```python
from build123d import *

# Parameters (mm, degrees)
SKETCH1_R                    = 3.429
BOSS_EXTRUDE1_DEPTH          = 165.1
SKETCH2_W                    = 12.954
SKETCH2_H                    = 12.954
CUT_EXTRUDE1_DEPTH           = 6.35
CUT_EXTRUDE1_DRAFT           = -45
CUT_EXTRUDE1_PROFILE_2_DEPTH = 6.35
CUT_EXTRUDE1_PROFILE_2_DRAFT = -45
CUT_EXTRUDE1_PROFILE_3_DEPTH = 6.35
CUT_EXTRUDE1_PROFILE_3_DRAFT = -45
SKETCH3_W                    = 6.35
SKETCH3_H                    = 12.7
CUT_EXTRUDE2_DEPTH           = 1.651


with BuildPart() as part:
    # Sketch1 → Boss-Extrude1 (new body)
    with BuildSketch(Plane.XY):
        with BuildLine():
            Line((-49.2125, 0), (-74.6125, 0))
            Line((-74.6125, 0), (-74.6125, -76.2))
            Line((-74.6125, -76.2), (74.6125, -76.2))
            Line((74.6125, -76.2), (74.6125, 0))
            Line((74.6125, 0), (49.2125, 0))
            ThreePointArc((49.2125, 0), (0, -49.2125), (-49.2125, 0))
        make_face()
        with Locations((-55.5625, -57.15)):
            Circle(SKETCH1_R, mode=Mode.SUBTRACT)
        with Locations((55.5625, -57.15)):
            Circle(SKETCH1_R, mode=Mode.SUBTRACT)
    extrude(amount=BOSS_EXTRUDE1_DEPTH)


with BuildPart() as cut_extrude1_tool:
    # Sketch2 → Cut-Extrude1 (with draft: the straight prism first)
    with BuildSketch(Plane(origin=(0, 0, 0), x_dir=(-1, 0, 0), z_dir=(0, 0, -1))):
        with Locations((-61.9125, -19.05)):
            Rectangle(SKETCH2_W, SKETCH2_H)
    extrude(amount=-CUT_EXTRUDE1_DEPTH)
    # Cut-Extrude1: the draft: its side faces are tilted about the plane it starts from
    cut_extrude1_sides = [cut_extrude1_tool.faces().sort_by_distance(p)[0] for p in [
        (68.3895, -19.05, 3.175),
        (61.9125, -25.527, 3.175),
        (55.4355, -19.05, 3.175),
        (61.9125, -12.573, 3.175),
    ]]
    draft(cut_extrude1_sides, Plane(origin=(0, 0, 0), x_dir=(-1, 0, 0), z_dir=(0, 0, -1)), CUT_EXTRUDE1_DRAFT)


with BuildPart() as part_1:
    add(part.part)

    # Cut-Extrude1: cut by cut_extrude1_tool
    add(cut_extrude1_tool.part, mode=Mode.SUBTRACT)


with BuildPart() as cut_extrude1_profile_2_tool:
    # Sketch2 → Cut-Extrude1 profile 2 (with draft: the straight prism first)
    with BuildSketch(Plane(origin=(0, 0, 0), x_dir=(-1, 0, 0), z_dir=(0, 0, -1))):
        with Locations((0, -63.5)):
            Rectangle(SKETCH2_W, SKETCH2_H)
    extrude(amount=-CUT_EXTRUDE1_PROFILE_2_DEPTH)
    # Cut-Extrude1 profile 2: the draft: its side faces are tilted about the plane it starts from
    cut_extrude1_profile_2_sides = [cut_extrude1_profile_2_tool.faces().sort_by_distance(p)[0] for p in [
        (6.477, -63.5, 3.175),
        (0, -69.977, 3.175),
        (-6.477, -63.5, 3.175),
        (0, -57.023, 3.175),
    ]]
    draft(cut_extrude1_profile_2_sides, Plane(origin=(0, 0, 0), x_dir=(-1, 0, 0), z_dir=(0, 0, -1)), CUT_EXTRUDE1_PROFILE_2_DRAFT)


with BuildPart() as part_2:
    add(part_1.part)

    # Cut-Extrude1 profile 2: cut by cut_extrude1_profile_2_tool
    add(cut_extrude1_profile_2_tool.part, mode=Mode.SUBTRACT)


with BuildPart() as cut_extrude1_profile_3_tool:
    # Sketch2 → Cut-Extrude1 profile 3 (with draft: the straight prism first)
    with BuildSketch(Plane(origin=(0, 0, 0), x_dir=(-1, 0, 0), z_dir=(0, 0, -1))):
        with Locations((61.9125, -19.05)):
            Rectangle(SKETCH2_W, SKETCH2_H)
    extrude(amount=-CUT_EXTRUDE1_PROFILE_3_DEPTH)
    # Cut-Extrude1 profile 3: the draft: its side faces are tilted about the plane it starts from
    cut_extrude1_profile_3_sides = [cut_extrude1_profile_3_tool.faces().sort_by_distance(p)[0] for p in [
        (-55.4355, -19.05, 3.175),
        (-61.9125, -25.527, 3.175),
        (-68.3895, -19.05, 3.175),
        (-61.9125, -12.573, 3.175),
    ]]
    draft(cut_extrude1_profile_3_sides, Plane(origin=(0, 0, 0), x_dir=(-1, 0, 0), z_dir=(0, 0, -1)), CUT_EXTRUDE1_PROFILE_3_DRAFT)


with BuildPart() as part_3:
    add(part_2.part)

    # Cut-Extrude1 profile 3: cut by cut_extrude1_profile_3_tool
    add(cut_extrude1_profile_3_tool.part, mode=Mode.SUBTRACT)

    # Sketch3 → Cut-Extrude2 (cut)
    with BuildSketch(Plane(origin=(0, 0, 0), x_dir=(1, 0, 0), z_dir=(0, 1, 0))):
        with Locations((71.4375, -19.05)):
            Rectangle(SKETCH3_W, SKETCH3_H)
        with Locations((71.4375, -57.15)):
            Rectangle(SKETCH3_W, SKETCH3_H)
        with Locations((71.4375, -95.25)):
            Rectangle(SKETCH3_W, SKETCH3_H)
        with Locations((71.4375, -133.35)):
            Rectangle(SKETCH3_W, SKETCH3_H)
        with Locations((-71.4375, -57.15)):
            Rectangle(SKETCH3_W, SKETCH3_H)
        with Locations((-71.4375, -95.25)):
            Rectangle(SKETCH3_W, SKETCH3_H)
        with Locations((-71.4375, -133.35)):
            Rectangle(SKETCH3_W, SKETCH3_H)
        with Locations((-71.4375, -19.05)):
            Rectangle(SKETCH3_W, SKETCH3_H)
    extrude(amount=-CUT_EXTRUDE2_DEPTH, mode=Mode.SUBTRACT)


solid = part_3.part
```
Can you work these out from the model? Positions are in its coordinate system, mm. A direction names the side the tool comes from. Coordinates: 2 decimals unless noted, no trailing zeros. Loops run counter-clockwise (first coordinate to the right, second up) from the corner with the lowest first, then second, coordinate; pieces in that order, holes last. Notation, with made-up numbers: (74.5, -32.75) -> (130.5, -32.75) arc R21 cw to (130.5, -11.75) -> close; hole circle Ø6 at (-37.5, 75.25). An arc over 180 degrees is marked (long way). Put each result on its own line as item: value. Start each with the question number.
Q1. I'm going to push flat-ended pins straight in: P1, Ø3, axis at x = -71.5, z = 21, coming from the +Y side; P2, Ø0.5, axis at y = -0.5, z = 136.5, coming from the +X side; P3, Ø3, axis at x = -44, y = -13, coming from the -Z side; P4, Ø8, axis at x = 30, z = 145, coming from the +Y side. Where does each tip first touch, or does it pass through?
Q2. I want a section at B-B (y = -16.5). Write out the boundary of the cut face in (x, z), plus the area to 3 significant figures.
Q3. Thinking about a two-plate mould opening in X: for faces 5 (the face through (57.86, -19.141, 2.425)), 6 (the face through (74.612, -39, 81)), 7 (the face through (71, -1.651, 95)), which applies, pulls with the +X half, pulls with the -X half, needs draft (parallel to the pull), parting line crosses it, or undercut?
Q4. For faces 1 (the face through (-61.822, -14.998, 2.425)), 2 (the face through (-52.3, -56.1, 81.4)), 3 (the face through (71, -1.651, 133)), 4 (the face through (-71, -1.651, 57)), which set-ups out of +Z, -Z, +X, -X, +Y, -Y let a thin tool reach every point of the face, with its end or its side?
Q5. If I drill on line 1 (X direction, y = -57, z = 41); line 2 (X direction, y = -54, z = 144); line 3 (Y direction, x = 56.5, z = 157.5), over which ranges is the centre line in solid material (lowest first)? Write a range as [from, to].
Q6. I want a section at D-D (y = -47). Write out the boundary of the cut face in (x, z).
Q7. I want a section at A-A (z = 70). Count the separate pieces of the cut face and the enclosed holes in it, plus the area to 3 significant figures.
Taken from the geometry:
1. P1: stops at y = -1.65
1. P2: stops at x = 68.26
1. P3: passes through
1. P4: stops at y = -35.58
2. outline: (-74.61, 0) -> (-68.39, 0) -> (-64.46, 3.93) -> (-59.36, 3.93) -> (-55.44, 0) -> (-46.36, 0) -> (-46.36, 165.1) -> (-74.61, 165.1) -> close; (46.36, 0) -> (55.44, 0) -> (59.36, 3.93) -> (64.46, 3.93) -> (68.39, 0) -> (74.61, 0) -> (74.61, 165.1) -> (46.36, 165.1) -> close
2. area: 9,260 mm2
3. face 5: undercut
3. face 6: pulls with the +X half
3. face 7: needs draft
4. face 1: -Z
4. face 2: +Z, -Z
4. face 3: +X, +Y
4. face 4: -X, +Y
5. line 1: x = [-74.61, -58.99], [-52.14, 52.14], [58.99, 74.61]
5. line 2: x = [-74.61, -56.92], [-54.21, 54.21], [56.92, 74.61]
5. line 3: y = [-76.2, -60.45], [-53.85, 0]
6. outline: (-74.61, 0) -> (-14.59, 0) -> (-14.59, 165.1) -> (-74.61, 165.1) -> close; (14.59, 0) -> (74.61, 0) -> (74.61, 165.1) -> (14.59, 165.1) -> close
7. separate pieces: 1
7. enclosed holes: 2
7. area: 7,490 mm2
